Autodesk Inventor part; units mm, degrees
ref_plane "YZ Plane" through (0, 0, 0) normal (1, 0, 0) x (0, 1, 0)
ref_plane "XZ Plane" through (0, 0, 0) normal (0, 1, 0) x (-1, 0, 0)
ref_plane "XY Plane" through (0, 0, 0) normal (0, 0, 1) x (1, 0, 0)
sketch "Sketch1" plane through (0, 0, 0) normal (0, 1, 0) x (-1, 0, 0)
  line L0 (0, 0) -> (19.05, 0)
  line L1 (19.05, 0) -> (19.05, -19.05)
  line L2 (19.05, -19.05) -> (0, -19.05)
  line L3 (0, -19.05) -> (0, 0)
  dimension "d0" = 19.05
  dimension "d1" = 19.05
extrude "Extrusion1" add sketch "Sketch1" along normal blind 76.2
sketch "Sketch4" plane through (-19.05, 0, 0) normal (0, 0, 1) x (1, 0, 0)
  circle A0 centre (9.525, 50.8) radius 3.175
  line L0 (0, 76.2) -> (19.05, 76.2)
  line L1 (19.05, 0) -> (19.05, 76.2)
  circle A1 centre (9.525, 25.4) radius 3.175
  line L2 (0, 0) -> (19.05, 0)
  dimension "d19" = 6.35
  dimension "d20" = 25.4
  dimension "d21" = 9.525
  dimension "d22" = 6.35
  dimension "d23" = 9.525
  dimension "d24" = 25.4
extrude "Extrusion4" cut sketch "Sketch4" against normal blind 25.4
sketch "Sketch5" plane through (0, 0, 0) normal (1, 0, 0) x (0, 0, -1)
  circle A0 centre (9.5599, 63.5) radius 3.175
  line L0 (0, 76.2) -> (19.05, 76.2)
  circle A1 centre (9.525, 38.1) radius 3.175
  line L1 (19.05, 0) -> (19.05, 76.2)
  circle A2 centre (9.525, 12.7) radius 3.175
  line L2 (0, 0) -> (19.05, 0)
  line L3 (0, 0) -> (0, 76.2)
  dimension "d27" = 6.35
  dimension "d28" = 12.7
  dimension "d29" = 6.35
  dimension "d30" = 9.525
  dimension "d31" = 38.1
  dimension "d32" = 6.35
  dimension "d33" = 12.7
  dimension "d34" = 9.525
extrude "Extrusion5" cut sketch "Sketch5" against normal blind 25.4 contours A0 | A1 | A2
properties part number "Experimental Block Bracket" material "Aluminum 6061"
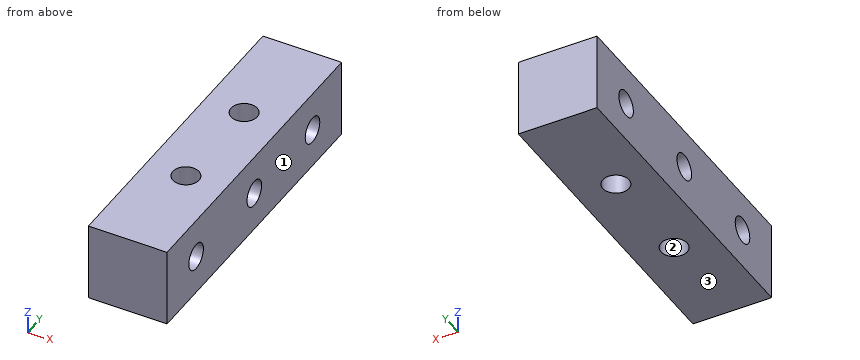
Work out the finished part from the listing and answer in its coordinate system (mm). Face numbers are marked on the shaded views. Give positions to 0.01 mm unless a question says otherwise; leave off trailing zeros. Write each loop counter-clockwise with the first axis right and the second up, starting at its lowest first coordinate (ties: lowest second). Pieces come first, ordered by that corner, then holes. Notation, with made-up numbers: (63.5, -17.75) - (102.5, -17.75) arc R33 cw to (102.5, 16.25) - close; hole circle Ø8 at (10, 59.5). An arc over 180 degrees is marked (long way). Use one line per item in the form item = value.
1. Determine the mould class of the marked faces 1, 2 and 3 for opening direction X: released by +X, released by -X, zero draft, split by the parting line, or undercut.
Filled in:
face_1 = released by +X
face_2 = undercut
face_3 = zero draft
2. A cutting plane is placed at D-D (y = 62.5). Write down the section's boundary in (x, z).
Filled in:
outline = (-19.05, -19.05) - (0, -19.05) - (0, -12.57) - (-19.05, -12.57) - close; (-19.05, -6.55) - (0, -6.55) - (0, 0) - (-19.05, 0) - close
3. Consider L1, parallel to Y at x = -4.5, z = -8; L2, parallel to Y at x = -7, z = -12; L3, parallel to Y at x = -5, z = -10.75. Determine where each line is inside the solid, lowest interval first.
Filled in:
L1 = 0 to 9.92, 15.48 to 35.32, 40.88 to 60.73, 66.27 to 76.2
L2 = 0 to 10.71, 14.69 to 23.48, 27.32 to 36.11, 40.09 to 48.88, 52.72 to 61.47, 65.53 to 76.2
L3 = 0 to 9.77, 15.63 to 35.17, 41.03 to 60.56, 66.44 to 76.2
4. A cutting plane is placed at C-C (z = -15). Write down the section's boundary in (x, y) (3 decimals), and give its area (3 significant figures).
Filled in:
outline = (-19.05, 0) - (0, 0) - (0, 76.2) - (-19.05, 76.2) - close; hole circle Ø6.35 at (-9.525, 25.4); hole circle Ø6.35 at (-9.525, 50.8)
area = 1,390 mm^2
5. A cutting plane is placed at B-B (y = 12.7). Write down the section's boundary in (x, z), and give its area (3 significant figures).
Filled in:
outline = (-19.05, -19.05) - (0, -19.05) - (0, -12.7) - (-19.05, -12.7) - close; (-19.05, -6.35) - (0, -6.35) - (0, 0) - (-19.05, 0) - close
area = 242 mm^2
6. This flat-tipped pin is pushed along its axis until it touches: pin 1 Ø5.5 at (x, y) = (-9.525, 50.8) entering from +Z. Where does it stop, or does it pass through?
Filled in:
pin_1 = through
7. A cutting plane is placed at A-A (x = -13.5). Write down the section's boundary in (y, z) (3 decimals).
Filled in:
outline = (0, -19.05) - (76.2, -19.05) - (76.2, 0) - (0, 0) - close; hole circle Ø6.35 at (12.7, -9.525); hole circle Ø6.35 at (38.1, -9.525); hole circle Ø6.35 at (63.5, -9.56)
